from build123d import *

# Parameters (mm, degrees)
SKETCH1_R                        = 49.4665
BOSS_EXTRUDE1_DEPTH              = 6.35
M3_SCREW_HOLE_3_0MM_DOWEL_HOLE_D = 3
SKETCH6_R                        = 3.429
CUT_EXTRUDE2_DEPTH               = 7.35
SKETCH7_R                        = 11.43
CUT_EXTRUDE3_DEPTH               = 7.35
SKETCH5_R                        = 3.429
CUT_EXTRUDE4_DEPTH               = 7.35
SKETCH11_R                       = 3.429
CUT_EXTRUDE7_DEPTH               = 7.35


with BuildPart() as part:
    # Sketch1 → Boss-Extrude1 (new body)
    with BuildSketch(Plane.XY):
        Circle(SKETCH1_R)
    extrude(amount=BOSS_EXTRUDE1_DEPTH)

    # M3 Screw Hole - Ø3.0mm Dowel Hole (through all)
    with Locations(Plane.XY.offset(6.35)):
        with Locations((0, 6.70774596), (-21.94774596, -15.24), (0, -37.18774596), (21.94774596, -15.24)):
            Hole(M3_SCREW_HOLE_3_0MM_DOWEL_HOLE_D / 2)

    # Sketch6 → Cut-Extrude2 (cut, through all)
    with BuildSketch(Plane.XY.offset(6.35)):
        with Locations((0, 38.128211777)):
            Circle(SKETCH6_R)
        with Locations((-33.02, -19.064105889)):
            Circle(SKETCH6_R)
        with Locations((33.02, -19.064105889)):
            Circle(SKETCH6_R)
    extrude(amount=-CUT_EXTRUDE2_DEPTH, mode=Mode.SUBTRACT)

    # Sketch7 → Cut-Extrude3 (cut, through all)
    with BuildSketch(Plane.XY.offset(6.35)):
        with Locations((0, -15.24)):
            Circle(SKETCH7_R)
    extrude(amount=-CUT_EXTRUDE3_DEPTH, mode=Mode.SUBTRACT)

    # Sketch5 → Cut-Extrude4 (cut, through all)
    with BuildSketch(Plane.XY.offset(6.35)):
        with Locations((0, 17.78)):
            Circle(SKETCH5_R)
    extrude(amount=-CUT_EXTRUDE4_DEPTH, mode=Mode.SUBTRACT)

    # Sketch11 → Cut-Extrude7 (cut, through all)
    with BuildSketch(Plane.XY.offset(6.35)):
        with Locations((19.38971276, -38.135544915)):
            Circle(SKETCH11_R)
    extrude(amount=-CUT_EXTRUDE7_DEPTH, mode=Mode.SUBTRACT)


solid = part.part
Check sheet for the modelled part. Datum: model origin and axes. Units: mm. Give positions to 0.01 mm unless a question says otherwise; leave off trailing zeros. Write each loop counter-clockwise with the first axis right and the second up, starting at its lowest first coordinate (ties: lowest second). Pieces come first, ordered by that corner, then holes. Notation, with made-up numbers: (42, 44) -> (65, 44) arc R13 cw to (65, 64) -> close; hole circle Ø10 at (-18.5, 20). An arc over 180 degrees is marked (long way). One line per item, written item: value. Start each with the question number.
Item 1: Material ranges on probe 1 along Y at (x, z) = (-1, 1.25); probe 2 along Y at (x, z) = (33.02, 2.5); probe 3 along Y at (x, z) = (-30, 1), recorded low to high. Write a range as from..to.
Item 2: Section check B-B on y = -6.5. Record the cut outline in (x, z).
Item 3: Section check D-D on z = 3.75. State how many separate pieces and enclosed holes the cut face has, then the cut area to 3 significant figures.
Item 4: Draft check along X on faces 1 (the flat face through (-1, 1, 0)), 2 (the cylindrical face through (47.18, 14.86, 3.13)), 3 (the cylindrical face through (20.56, -15.81, 3.13)). Enter one of: +X half, -X half, draft (parallel to the pull), parting line (faces both ways), or undercut.
Item 5: Section check A-A on x = 0. Record the cut outline in (y, z), then the cut area to 3 significant figures.
Item 6: Gauge pin test, flat ends, axial feed: pin 1 (2 mm diameter, centred on x = -18.5, z = 4.5, fed in from -Y); pin 2 (4 mm diameter, centred on x = 0, y = 17.78, fed in from -Z); pin 3 (2 mm diameter, centred on y = -2, z = 2, fed in from -X); pin 4 (1.5 mm diameter, centred on x = -19, z = 1, fed in from +Y). Record the tip position at first contact, or that the pin passes through.
Item 7: Section check C-C on y = -20.5. Record the cut outline in (x, z), then the cut area to 3 significant figures.
Results list:
1. probe 1: -49.46..-38.31, -36.07..-26.63, -3.85..5.59, 7.83..14.5, 21.06..34.85, 41.41..49.46
1. probe 2: -36.83..-22.49, -15.64..36.83
1. probe 3: -39.33..-20.69, -17.44..39.33
2. outline: (-49.04, 0) -> (-7.37, 0) -> (-7.37, 6.35) -> (-49.04, 6.35) -> close; (7.37, 0) -> (49.04, 0) -> (49.04, 6.35) -> (7.37, 6.35) -> close
3. separate pieces: 1
3. enclosed holes: 10
3. area: 7,060 mm²
4. face 1: draft
4. face 2: parting line
4. face 3: undercut
5. outline: (-49.47, 0) -> (-38.69, 0) -> (-38.69, 6.35) -> (-49.47, 6.35) -> close; (-35.69, 0) -> (-26.67, 0) -> (-26.67, 6.35) -> (-35.69, 6.35) -> close; (-3.81, 0) -> (5.21, 0) -> (5.21, 6.35) -> (-3.81, 6.35) -> close; (8.21, 0) -> (14.35, 0) -> (14.35, 6.35) -> (8.21, 6.35) -> close; (21.21, 0) -> (34.7, 0) -> (34.7, 6.35) -> (21.21, 6.35) -> close; (41.56, 0) -> (49.47, 0) -> (49.47, 6.35) -> (41.56, 6.35) -> close
5. area: 358 mm²
6. pin 1: y = -46.27
6. pin 2: through
6. pin 3: x = -49.46
6. pin 4: y = 45.98
7. outline: (-45.02, 0) -> (-36.13, 0) -> (-36.13, 6.35) -> (-45.02, 6.35) -> close; (-29.91, 0) -> (-10.15, 0) -> (-10.15, 6.35) -> (-29.91, 6.35) -> close; (10.15, 0) -> (29.91, 0) -> (29.91, 6.35) -> (10.15, 6.35) -> close; (36.13, 0) -> (45.02, 0) -> (45.02, 6.35) -> (36.13, 6.35) -> close
7. area: 364 mm²
